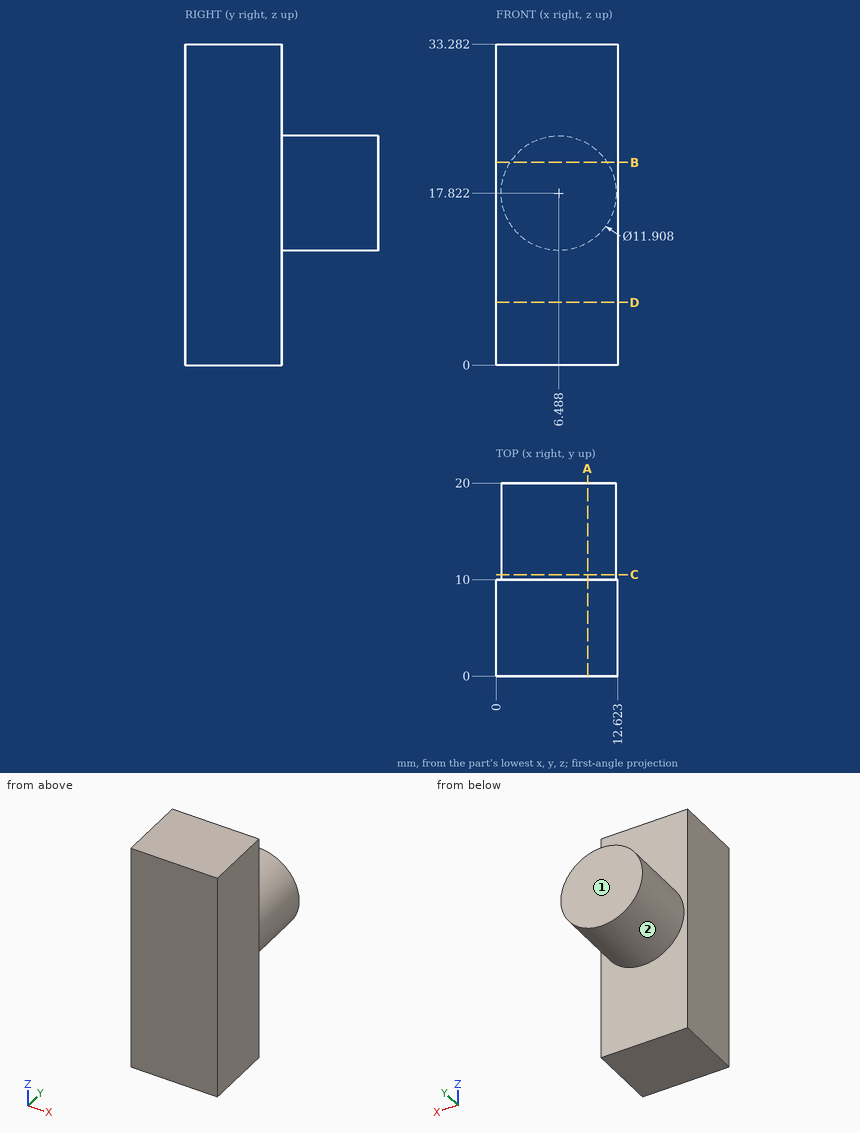
The figure shows three views and two pictorial views of one solid part (mm, origin at its lowest corner). Answer the questions. A direction names the side the tool comes from. Round coordinates to 2 decimals unless told otherwise and drop trailing zeros. Loops run counter-clockwise (first coordinate to the right, second up) from the corner with the lowest first, then second, coordinate; pieces in that order, holes last. Notation, with made-up numbers: M -15,2 L 7,2 A7 cw 7,9 Z; hole C 42,-31 d6. An arc over 180 degrees is marked long. Return JSON: item names as keys, results as strings.
Q1. Which of the six approach directions +Z, -Z, +X, -X, +Y, -Y give full straight-line access (tool end or side, diameter ignored) to the marked faces 1 and 2?
Results list:
{"face 1": "+Z, -Z, +X, -X, +Y", "face 2": "+Y"}
Q2. Find section C-C, the plane y = 10.5. Determine the outline of the cut face in (x, z) (1 decimal).
Results list:
{"outline": "C 6.5,17.8 d11.9"}
Q3. Find the intervals of material crossed by line 1 along Y through (x, z) = (1.75, 4); line 2 along Z through (x, y) = (6.25, 19); line 3 along X through (y, z) = (13.75, 16) (1 decimal), in increasing order. Write a range as from..to.
Results list:
{"line 1": "y = 0..10", "line 2": "z = 11.87..23.77", "line 3": "x = 0.8..12.2"}
Q4. Find section B-B, the plane z = 21. Determine the outline of the cut face in (x, y).
Results list:
{"outline": "M 0,0 L 12.62,0 L 12.62,10 L 11.52,10 L 11.52,20 L 1.45,20 L 1.45,10 L 0,10 Z"}
Q5. Each of these flat-tipped pins is pushed along its axis until it touches: pin 1 Ø8 at (y, z) = (15, 21) entering from -X; pin 2 Ø2 at (y, z) = (17, 12.5) entering from +X (1 decimal); pin 3 Ø5 at (x, y) = (6.5, 15) entering from -Z. Where does it stop, or does it pass through?
Results list:
{"pin 1": "stops at x = 0.53", "pin 2": "stops at x = 10.6", "pin 3": "stops at z = 11.87"}
Q6. Find section A-A, the plane x = 9.5. Determine the outline of the cut face in (y, z) (1 decimal).
Results list:
{"outline": "M 0,0 L 10,0 L 10,12.7 L 20,12.7 L 20,23 L 10,23 L 10,33.3 L 0,33.3 Z"}
Q7. Find section D-D, the plane z = 6.5. Determine the outline of the cut face in (x, y), plus the area to 3 significant figures.
Results list:
{"outline": "M 0,0 L 12.62,0 L 12.62,10 L 0,10 Z", "area": "126 mm2"}
